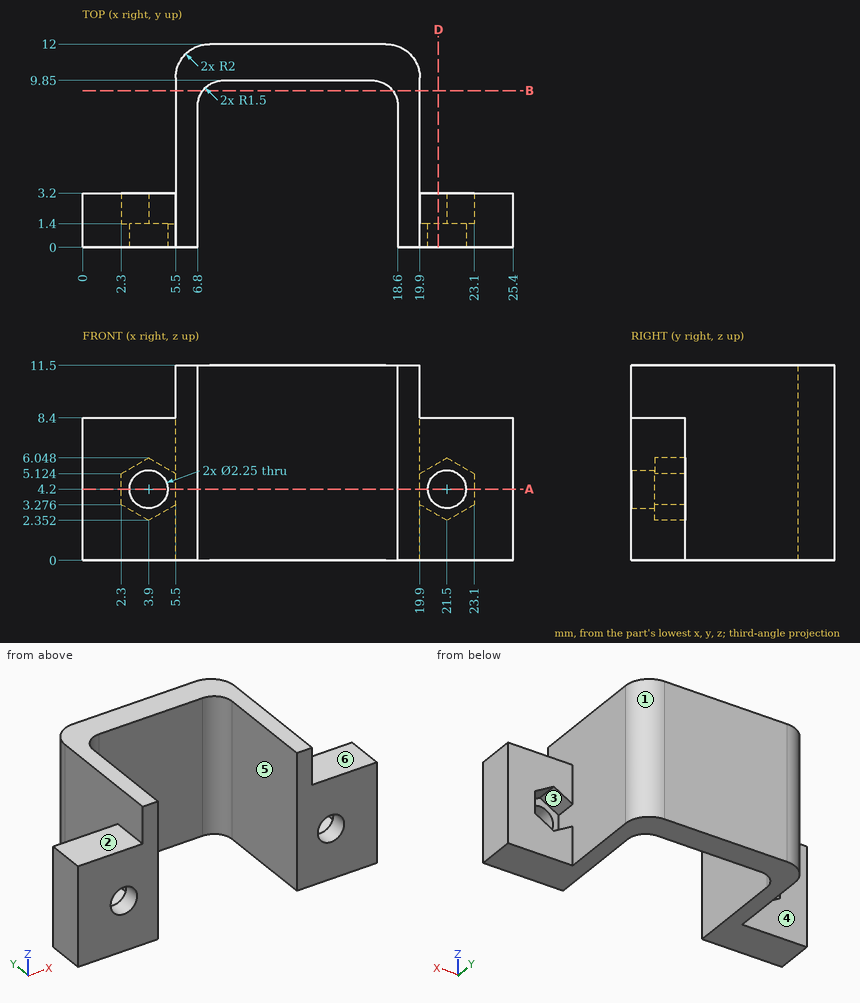
Input: dimensioned drawing with shaded views. Units: mm. Origin: part minimum x, y, z. A direction names the side the tool comes from. Give positions to 0.01 mm unless a question says otherwise; leave off trailing zeros. Order: outer loops, then holes, each group sorted by start corner. A loop starts at its lowest first (then second) coordinate and runs counter-clockwise, first axis right, second up. Notation, with made-up numbers: (1.25, -32.5) -> (19.25, -32.5) arc R29 ccw to (19.25, -2.5) -> close; hole circle Ø10 at (81, 50.5). An arc over 180 degrees is marked (long way). Use one line per item in the form item = value.
1) Section A-A, the plane z = 4.2. Count the separate pieces of the cut face and the enclosed holes in it.
Response values:
separate_pieces = 3
enclosed_holes = 0
2) Section B-B, the plane y = 9.25. Return loops of the section in (x, z).
Response values:
outline = (5.5, 0) -> (7.1, 0) -> (7.1, 11.5) -> (5.5, 11.5) -> close; (18.3, 0) -> (19.9, 0) -> (19.9, 11.5) -> (18.3, 11.5) -> close
3) First-contact query: pin 1 Ø1.5 at (x, y) = (17, 4) entering from +Z; pin 2 Ø4.5 at (x, z) = (13.5, 7.5) entering from -Y; pin 3 Ø3 at (x, z) = (3.5, 2.5) entering from +Y; pin 4 Ø0.9 at (y, z) = (2.5, 4.5) entering from -X. Flat tips, straight axial feed; report the tip coordinate or a pass-through.
Response values:
pin_1 = through
pin_2 = 9.85
pin_3 = 3.2
pin_4 = 0
4) Line query: probe 1 along X at (y, z) = (0.6, 4.2) (1 decimal); probe 2 along Z at (x, y) = (21.5, 0.6) (1 decimal); probe 3 along X at (y, z) = (7.75, 9.5). Output: solid intervals per line, ascending.
Response values:
probe_1 = 0 to 2.8, 5 to 6.8, 18.6 to 20.4, 22.6 to 25.4
probe_2 = 0 to 3.1, 5.3 to 8.4
probe_3 = 5.5 to 6.8, 18.6 to 19.9
5) Section D-D, the plane x = 21. Return loops of the section in (y, z).
Response values:
outline = (0, 0) -> (3.2, 0) -> (3.2, 2.64) -> (1.4, 2.64) -> (1.4, 3.19) -> (0, 3.19) -> close; (0, 5.21) -> (1.4, 5.21) -> (1.4, 5.76) -> (3.2, 5.76) -> (3.2, 8.4) -> (0, 8.4) -> close
6) Mould query, pull axis Z, two halves, no side actions, for the marked faces 1, 2 and 3. Classes: pulls with the +Z half, pulls with the -Z half, needs draft (parallel to the pull), parting line crosses it, or undercut.
Response values:
face_1 = needs draft
face_2 = pulls with the +Z half
face_3 = undercut
7) Reachability of the marked faces 4, 5 and 6 from +Z, -Z, +X, -X, +Y, -Y: full face, straight path, thin tool, end or side. Return the list, or none.
Response values:
face_4 = +Z, -Z, -X, +Y
face_5 = +Z, -Z, -Y
face_6 = +Z, +X, +Y, -Y
